```python
from build123d import *

# Parameters (mm, degrees)
EXTRUDE_DEPTH     = 4.83
CYLINDER002_R     = 11
CYLINDER002_DEPTH = 28.19


with BuildPart() as extrude_body:
    # Sketch → Extrude (new body)
    with BuildSketch(Plane.XY):
        Polygon((12.25, -7.072541), (12.25, 7.072541), (0, 14.145082), (-12.25, 7.072541), (-12.25, -7.072541), (0, -14.145082), align=None)
    extrude(amount=EXTRUDE_DEPTH)


with BuildPart() as extrude_body_1:
    # Extrude placement: moved
    add(extrude_body.part.moved(Location((0, 0, 12.19))))


with BuildPart() as powerplug:
    # Cylinder002 → Cylinder002 (new body)
    with BuildSketch(Plane.XY):
        Circle(CYLINDER002_R)
    extrude(amount=CYLINDER002_DEPTH)

    # Fusion: union Extrude body
    add(extrude_body_1.part)


with BuildPart() as powerplug_1:
    # Fusion placement: moved
    add(powerplug.part.moved(Location((-40, 25, -147))))


solid = powerplug_1.part
```
Model file for the job. Use its own axes, mm. A direction names the side the tool comes from. Coordinates: 2 decimals unless noted, no trailing zeros. Write each loop counter-clockwise with the first axis right and the second up, starting at its lowest first coordinate (ties: lowest second). Pieces come first, ordered by that corner, then holes. Notation, with made-up numbers: (38.25, -15) - (68.25, -15) arc R27 ccw to (68.25, 19) - close; hole circle Ø9 at (19, 84.25). An arc over 180 degrees is marked (long way). Use a Markdown table: item, result. Add a question column.
Item 1: Band-saw the part on B-B, the plane x = -49.75. Write the cut outline in (y, z).
Item 2: Drop flat-ended pins along their axis: pin 1 (2 mm diameter, centred on x = -32, z = -124.5, fed in from +Y); pin 2 (6 mm diameter, centred on y = 14, z = -121.5, fed in from +X); pin 3 (3 mm diameter, centred on x = -39, z = -124.5, fed in from +Y). Give the stop position or say it passes through.
Item 3: Band-saw the part on A-A, the plane y = 25. Write the cut outline in (x, z), and give its area (3 significant figures).
Item 4: Drill centre lines: line 1 along Z through (x, y) = (-31, 33.25); line 2 along Y through (x, z) = (-41.75, -142.5); line 3 along Y through (x, z) = (-49.5, -130.5). Where is each one in solid material? Low to high.
Item 5: 3-axis set-ups, long thin cutter, end or side, ignore diameter. For faces 1 (the face through (-29.839, 20.787, -124.473)), 2 (the face through (-51, 23, -134.81)), 3 (the face through (-27.75, 25, -132)): which of +Z, -Z, +X, -X, +Y, -Y reach the whole face in a straight line?
Item 6: Band-saw the part on C-C, the plane z = -136.5. Write the cut outline in (x, y).
Item 7: Band-saw the part on D-D, the plane y = 37. Write the cut outline in (x, z).
A:
| question | item | result |
|---|---|---|
| 1 | outline | (16.48, -134.81) - (19.91, -134.81) - (19.91, -147) - (30.09, -147) - (30.09, -134.81) - (33.52, -134.81) - (33.52, -129.98) - (30.09, -129.98) - (30.09, -118.81) - (19.91, -118.81) - (19.91, -129.98) - (16.48, -129.98) - close |
| 2 | pin 1 | stops at y = 33.49 |
| 2 | pin 2 | stops at x = -32.45 |
| 2 | pin 3 | stops at y = 36 |
| 3 | outline | (-52.25, -134.81) - (-51, -134.81) - (-51, -147) - (-29, -147) - (-29, -134.81) - (-27.75, -134.81) - (-27.75, -129.98) - (-29, -129.98) - (-29, -118.81) - (-51, -118.81) - (-51, -129.98) - (-52.25, -129.98) - close |
| 3 | area | 632 mm² |
| 4 | line 1 | z = -134.81 to -129.98 |
| 4 | line 2 | y = 14.14 to 35.86 |
| 4 | line 3 | y = 16.34 to 33.66 |
| 5 | face 1 | +Z |
| 5 | face 2 | -Z |
| 5 | face 3 | +Z, -Z, +X, +Y, -Y |
| 6 | outline | circle Ø22 at (-40, 25) |
| 7 | outline | (-43.72, -134.81) - (-36.28, -134.81) - (-36.28, -129.98) - (-43.72, -129.98) - close |
